Build history of the part. All positions in model axes, mm. A direction names the side the tool comes from. Coordinates: 2 decimals unless noted, no trailing zeros. Write each loop counter-clockwise with the first axis right and the second up, starting at its lowest first coordinate (ties: lowest second). Pieces come first, ordered by that corner, then holes. Notation, with made-up numbers: (-30.75, 45) -> (28.25, 45) arc R24 cw to (28.25, 77) -> close; hole circle Ø8 at (-17.75, 1). An arc over 180 degrees is marked (long way). Write each question's results on one line, items separated by ' | '. Start each with the question number.
Q1. Drop flat-ended pins along their axis: pin 1 Ø1 at (x, y) = (2, -50) entering from -Z; pin 2 Ø1 at (x, z) = (1.5, -71.5) entering from -Y; pin 3 Ø1 at (x, y) = (1, -50.5) entering from +Z. Give the stop position or say it passes through.
Q2. Tool access for faces 5 (the face through (2, -48.458, -70)), 6 (the face through (2, -48.458, -6)), 7 (the face through (1.565, -47.283, 39.366)): list every direction of +Z, -Z, +X, -X, +Y, -Y with a clear straight run to the whole face (end or side of a thin tool).
Q3. Two-plate mould, pull along Z, no slides. Class faces 1 (the face through (2, -50, 0)), 2 (the face through (2, -50, 38.1)), 3 (the face through (2, -51.633, -19)), 4 (the face through (2, -45, -55.88)): released by +Z, released by -Z, zero draft, split by the parting line, or undercut.
Q4. Saw through at B-B on y = -12.5. Give the cut face in (x, z) (3 decimals).
Q5. Drill centre lines: line 1 (Z direction, x = 1.6, y = 6.5); line 2 (Z direction, x = 1.1, y = -17); line 3 (Y direction, x = 0.65, z = -7.5). Where is each one in solid material? Low to high.
Q6. Saw through at A-A on x = 1.75. Give the cut face in (y, z), and give its area (3 significant figures).
Q7. Saw through at C-C on z = -5. Give the cut face in (x, y) (3 decimals).
from build123d import *

# Parameters (mm, degrees)
F0_W     = 3.175
F0_H     = 12.7
F1_DEPTH = 3.175


with BuildPart() as f1:
    # F0 (on Right) → F1 (new body)
    with BuildSketch(Plane.YZ):
        with BuildLine():
            ThreePointArc((-45.94075, 38.34122), (-47.308793, 39.364207), (-48.457631, 38.1))
            Line((-48.457631, 38.1), (-48.457631, 25.4))
            Line((-48.457631, 25.4), (-48.457631, 12.7))
            Line((-48.457631, 12.7), (-48.457631, 0))
            Line((-48.457631, 0), (-48.457631, -12.7))
            Line((-48.457631, -12.7), (-48.457631, -25.4))
            Line((-48.457631, -25.4), (-48.457631, -55.88))
            Line((-48.457631, -55.88), (-40.837631, -55.88))
            Line((-40.837631, -55.88), (-40.837631, -66.04))
            Line((-40.837631, -66.04), (-48.457631, -66.04))
            Line((-48.457631, -66.04), (-48.457631, -73.66))
            Line((-48.457631, -73.66), (-40.837631, -73.66))
            Line((-40.837631, -73.66), (63.302369, -73.66))
            Line((63.302369, -73.66), (65.830783, -73.66))
            ThreePointArc((65.830783, -73.66), (65.17357, -71.959562), (63.543589, -71.143119))
            ThreePointArc((63.543589, -71.143119), (-7.961537, -33.163906), (-45.94075, 38.34122))
        make_face()
        with Locations((-50.045131, 31.75)):
            Rectangle(F0_W, F0_H)
        with Locations((-50.045131, 6.35)):
            Rectangle(F0_W, F0_H)
        with Locations((-50.045131, -19.05)):
            Rectangle(F0_W, F0_H)
    extrude(amount=F1_DEPTH)


solid = f1.part
Returned:
1) pin 1: stops at z = -25.4 | pin 2: stops at y = -48.46 | pin 3: stops at z = 38.1
2) face 5: -Z, +X, -X, -Y | face 6: +X, -X, -Y | face 7: +Z, +X, -X
3) face 1: undercut | face 2: released by +Z | face 3: zero draft | face 4: undercut
4) outline: (0, -73.66) -> (3.175, -73.66) -> (3.175, -28.404) -> (0, -28.404) -> close
5) line 1: z = -73.66 to -45.75 | line 2: z = -73.66 to -23.2 | line 3: y = -48.46 to -28.17
6) outline: (-51.63, -25.4) -> (-48.46, -25.4) -> (-48.46, -55.88) -> (-40.84, -55.88) -> (-40.84, -66.04) -> (-48.46, -66.04) -> (-48.46, -73.66) -> (65.83, -73.66) arc R2.53 ccw to (63.54, -71.14) arc R138.26 cw to (-45.94, 38.34) arc R1.27 ccw to (-48.46, 38.1) -> (-51.63, 38.1) -> (-51.63, 25.4) -> (-48.46, 25.4) -> (-48.46, 12.7) -> (-51.63, 12.7) -> (-51.63, 0) -> (-48.46, 0) -> (-48.46, -12.7) -> (-51.63, -12.7) -> close | area: 4,110 mm2
7) outline: (0, -48.458) -> (3.175, -48.458) -> (3.175, -29.661) -> (0, -29.661) -> close
